from build123d import *

# Parameters (mm, degrees)
BOSS_EXTRUDE4_DEPTH = 5


with BuildPart() as part:
    # Sketch5 → Boss-Extrude4 (new body)
    with BuildSketch(Plane.XZ.offset(20.3)):
        Polygon((0, 100), (-62.613989109, 37.386010891), (-40.345458425, 24.089756452), (10.264785123, 74.7), (100, 74.7), (100, 100), align=None)
    extrude(amount=BOSS_EXTRUDE4_DEPTH)


solid = part.part
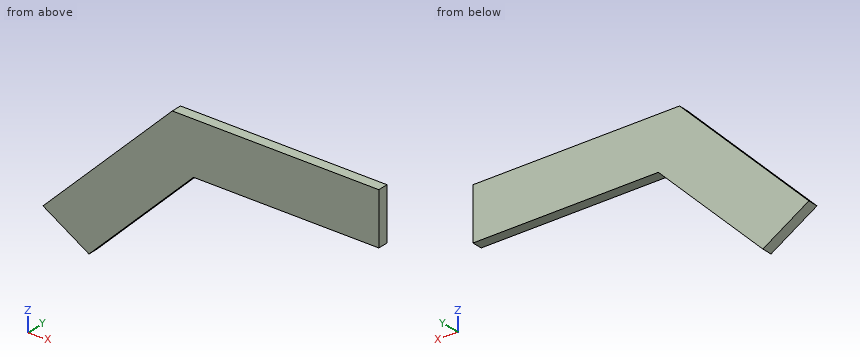
The listing builds one solid part. Answer for the finished solid, in the listing's coordinates (mm). Give positions to 0.01 mm unless a question says otherwise; leave off trailing zeros. Loops run counter-clockwise (first coordinate to the right, second up) from the corner with the lowest first, then second, coordinate; pieces in that order, holes last. Notation, with made-up numbers: (60, 59.5) - (115, 59.5) arc R23 ccw to (115, 94.5) - close; hole circle Ø9 at (86, -16). An arc over 180 degrees is marked (long way). Answer as a JSON object with one key per item and string values.
1. Find the intervals of material crossed by L1, parallel to Z at x = 82, y = -22.9; L2, parallel to X at y = -21.45, z = 66.5; L3, parallel to X at y = -20.8, z = 33, in increasing order. Write a range as [from, to].
Determined:
{"L1": "[74.7, 100]", "L2": "[-33.5, 2.06]", "L3": "[-55.27, -31.44]"}
2. A cutting plane is placed at C-C (x = 20). Write down the section's boundary in (y, z), then the cut area to 4 significant figures.
Determined:
{"outline": "(-25.3, 74.7) - (-20.3, 74.7) - (-20.3, 100) - (-25.3, 100) - close", "area": "126.5 mm²"}
3. A cutting plane is placed at A-A (y = -23.35). Write down the section's boundary in (x, z).
Determined:
{"outline": "(-62.61, 37.39) - (-40.35, 24.09) - (10.26, 74.7) - (100, 74.7) - (100, 100) - (0, 100) - close"}
4. A cutting plane is placed at B-B (z = 92.5). Write down the section's boundary in (x, y), then the cut area to 4 significant figures.
Determined:
{"outline": "(-7.5, -25.3) - (100, -25.3) - (100, -20.3) - (-7.5, -20.3) - close", "area": "537.5 mm²"}
